Geometry: final body of the model. Coordinates: model frame, mm. Face numbers are marked on the shaded views. A direction names the side the tool comes from. Round coordinates to 2 decimals unless told otherwise and drop trailing zeros. Loops run counter-clockwise (first coordinate to the right, second up) from the corner with the lowest first, then second, coordinate; pieces in that order, holes last. Notation, with made-up numbers: (62.25, 4) - (120.25, 4) arc R22 cw to (120.25, 15) - close; hole circle Ø3 at (61.5, 0). An arc over 180 degrees is marked (long way). Return JSON: item names as keys, results as strings. Group by question number.
1. Section A-A on z = 164.5. Return loops of the section in (x, y).
2. Draft query along X for the marked faces 4 and 5. Return one class per face: +X half, -X half, draft (parallel to the pull), parting line (faces both ways), or undercut.
3. Material intervals for probe 1 along Z at (x, y) = (442, 35.5); probe 2 along X at (y, z) = (29.5, 139); probe 3 along X at (y, z) = (147.5, 135.5), sorted ascending.
4. Section C-C on x = 140.5. Return loops of the section in (y, z).
5. First-contact query: pin 1 Ø14.5 at (y, z) = (50, 9.5) entering from -X; pin 2 Ø8 at (y, z) = (26.5, 86.5) entering from +X; pin 3 Ø4 at (x, z) = (254.5, 243.5) entering from -Y. Flat tips, straight axial feed; report the tip coordinate or a pass-through.
6. Set-up query: the marked faces 1, 2 and 3. Return all of +Z, -Z, +X, -X, +Y, -Y with unobstructed straight access to the full face (end or side cutting, diameter ignored); none if empty.
7. Section D-D on x = 445. Return loops of the section in (y, z), and give its area (3 significant figures).
8. Section B-B on y = 120. Return loops of the section in (x, z).
from build123d import *

# Parameters (mm, degrees)
BOSS_EXTRUDE1_DEPTH = 250
SKETCH2_W           = 299.205309142
SKETCH2_H           = 220
CUT_EXTRUDE1_DEPTH  = 581.086200491
SKETCH4_W           = 299.205309142
SKETCH4_H           = 15
CUT_EXTRUDE2_DEPTH  = 20
SHELL1_START        = 2
SHELL1_DEPTH        = 246
SKETCH5_W           = 15
SKETCH5_H           = 20
BOSS_EXTRUDE2_DEPTH = 2
SKETCH6_W           = 15
SKETCH6_H           = 20
BOSS_EXTRUDE3_DEPTH = 2
SKETCH7_W           = 100
SKETCH7_H           = 120
BOSS_EXTRUDE4_DEPTH = 250
CUT_EXTRUDE3_DEPTH  = 100


# Read off the part's stored shape, not the designer's step: Shell1
with BuildPart() as part:
    # Sketch1 → Boss-Extrude1 (new body)
    with BuildSketch(Plane.XY):
        with BuildLine():
            Line((0, 0), (520, 0))
            ThreePointArc((520, 0), (502.285771516, 42.567121511), (459.602654571, 60))
            Line((459.602654571, 60), (60.397345429, 60))
            ThreePointArc((60.397345429, 60), (17.714228484, 42.567121511), (0, 0))
        make_face()
    extrude(amount=BOSS_EXTRUDE1_DEPTH)

    # Sketch2 → Cut-Extrude1 (cut, through all)
    with BuildSketch(Plane(origin=(0, 60, 0), x_dir=(1, 0, 0), z_dir=(0, 1, 0))):
        with Locations((260, -125)):
            Rectangle(SKETCH2_W, SKETCH2_H)
    extrude(amount=-CUT_EXTRUDE1_DEPTH, mode=Mode.SUBTRACT)

    # Sketch4 → Cut-Extrude2 (cut)
    with BuildSketch(Plane(origin=(0, 60, 0), x_dir=(1, 0, 0), z_dir=(0, 1, 0))):
        with Locations((260, -242.5)):
            Rectangle(SKETCH4_W, SKETCH4_H)
        with Locations((260, -7.5)):
            Rectangle(SKETCH4_W, SKETCH4_H)
    extrude(amount=-CUT_EXTRUDE2_DEPTH, mode=Mode.SUBTRACT)

    # Shell1 outline → Shell1 (cut)
    with BuildSketch(Plane.XY.offset(SHELL1_START)):
        with BuildLine():
            Line((110.397345429, 38), (110.397345429, 58))
            Line((110.397345429, 58), (60.390688921, 58))
            ThreePointArc((60.390688921, 58), (19.126088629, 41.15055453), (2, 0))
            Line((2, 0), (518, 0))
            ThreePointArc((518, 0), (500.873911371, 41.15055453), (459.609311079, 58))
            Line((459.609311079, 58), (409.602654571, 58))
            Line((409.602654571, 58), (409.602654571, 38))
            Line((409.602654571, 38), (110.397345429, 38))
        make_face()
    extrude(amount=SHELL1_DEPTH, mode=Mode.SUBTRACT)

    # Sketch5 → Boss-Extrude2 (add)
    with BuildSketch(Plane.ZY.offset(-409.602654571)):
        with Locations((7.5, 50)):
            Rectangle(SKETCH5_W, SKETCH5_H)
        with Locations((242.5, 50)):
            Rectangle(SKETCH5_W, SKETCH5_H)
    extrude(amount=BOSS_EXTRUDE2_DEPTH)

    # Sketch6 → Boss-Extrude3 (add)
    with BuildSketch(Plane(origin=(110.397345429, 0, 0), x_dir=(0, 0, -1), z_dir=(1, 0, 0))):
        with Locations((-242.5, 50)):
            Rectangle(SKETCH6_W, SKETCH6_H)
        with Locations((-7.5, 50)):
            Rectangle(SKETCH6_W, SKETCH6_H)
    extrude(amount=BOSS_EXTRUDE3_DEPTH)

    # Sketch7 → Boss-Extrude4 (add)
    with BuildSketch(Plane.XY.offset(250)):
        with Locations((260, 100)):
            Rectangle(SKETCH7_W, SKETCH7_H)
    extrude(amount=-BOSS_EXTRUDE4_DEPTH)

    # Sketch8 → Cut-Extrude3 (cut)
    with BuildSketch(Plane(origin=(310, 0, 0), x_dir=(0, 0, -1), z_dir=(1, 0, 0))):
        Polygon((-248, 145), (-2, 145), (-2, 40), (-15, 40), (-235, 40), (-248, 40), align=None)
    extrude(amount=-CUT_EXTRUDE3_DEPTH, mode=Mode.SUBTRACT)


solid = part.part
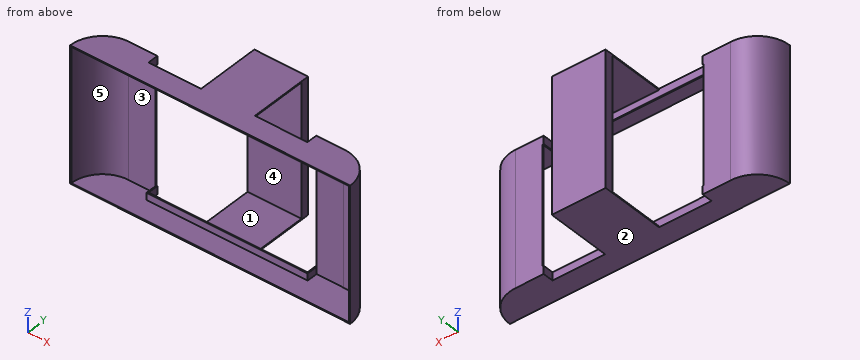
Taken from the geometry:
{
 "1": {"outline": "(0, 0) - (2, 0) arc R58 cw to (60.39, 58) - (110.4, 58) - (110.4, 60) - (60.4, 60) arc R60 ccw to start; (210, 145) - (310, 145) - (310, 160) - (210, 160) - close; (409.6, 58) - (459.61, 58) arc R58 cw to (518, 0) - (520, 0) arc R60 ccw to (459.6, 60) - (409.6, 60) - close"},
 "2": {"face 4": "draft", "face 5": "undercut"},
 "3": {"probe 1": "0 to 2, 248 to 250", "probe 2": "7.75 to 10.06, 509.94 to 512.25", "probe 3": "210 to 310"},
 "4": {"outline": "(0, 0) - (40, 0) - (40, 15) - (38, 15) - (38, 2) - (0, 2) - close; (0, 248) - (38, 248) - (38, 235) - (40, 235) - (40, 250) - (0, 250) - close"},
 "5": {"pin 1": "x = 17.9", "pin 2": "x = 515.62", "pin 3": "y = 38"},
 "6": {"face 1": "none", "face 2": "-Z, +X, -X, +Y, -Y", "face 3": "-Y"},
 "7": {"outline": "(0, 0) - (60, 0) - (60, 250) - (0, 250) - (0, 248) - (58, 248) - (58, 2) - (0, 2) - close", "area": "732 mm2"},
 "8": {"outline": "(210, 0) - (310, 0) - (310, 2) - (210, 2) - close; (210, 248) - (310, 248) - (310, 250) - (210, 250) - close"}
}
